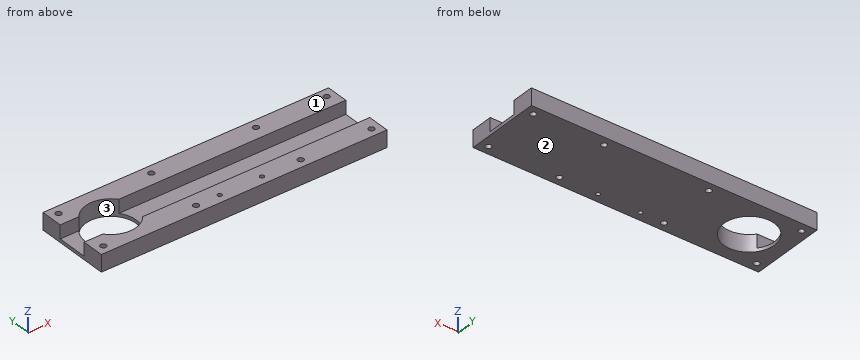
from build123d import *

# Parameters (mm, degrees)
F0_W     = 323.85
F0_H     = 85.09
F1_DEPTH = 19.05
F2_R     = 28.575
F3_DEPTH = 19.051
F4_R     = 3.302
F5_DEPTH = 19.051
F6_R     = 2.413
F7_DEPTH = 19.051
F9_DEPTH = 15.24


with BuildPart() as f1:
    # F0 (on Top) → F1 (new body)
    with BuildSketch(Plane.XY):
        with Locations((161.925, 42.545)):
            Rectangle(F0_W, F0_H)
    extrude(amount=F1_DEPTH)

    # F2 (on face) → F3 (cut, through all)
    with BuildSketch(Plane.XY.offset(19.05)):
        with Locations((43.815, 42.545)):
            Circle(F2_R)
    extrude(amount=-F3_DEPTH, mode=Mode.SUBTRACT)

    # F4 (on face) → F5 (cut, through all)
    with BuildSketch(Plane.XY.offset(19.05)):
        with Locations((9.906, 75.184)):
            Circle(F4_R)
        with Locations((115.062, 75.184)):
            Circle(F4_R)
        with Locations((233.68, 75.184)):
            Circle(F4_R)
        with Locations((313.944, 75.184)):
            Circle(F4_R)
        with Locations((115.062, 9.906)):
            Circle(F4_R)
        with Locations((9.906, 9.906)):
            Circle(F4_R)
        with Locations((233.68, 9.906)):
            Circle(F4_R)
        with Locations((313.944, 9.906)):
            Circle(F4_R)
    extrude(amount=-F5_DEPTH, mode=Mode.SUBTRACT)

    # F6 (on face) → F7 (cut, through all)
    with BuildSketch(Plane.XY.offset(19.05)):
        with Locations((141.859, 10.033)):
            Circle(F6_R)
        with Locations((189.865, 10.033)):
            Circle(F6_R)
    extrude(amount=-F7_DEPTH, mode=Mode.SUBTRACT)

    # F8 (on face) → F9 (cut)
    with BuildSketch(Plane.XY.offset(19.05)):
        with BuildLine():
            Line((323.85, 60.0075), (66.433393, 60.0075))
            ThreePointArc((66.433393, 60.0075), (70.859881, 51.770238), (72.39, 42.545))
            ThreePointArc((72.39, 42.545), (70.859881, 33.319762), (66.433393, 25.0825))
            Line((66.433393, 25.0825), (323.85, 25.0825))
            Line((323.85, 25.0825), (323.85, 60.0075))
        make_face()
        with BuildLine():
            Line((21.196607, 60.0075), (0, 60.0075))
            Line((0, 60.0075), (0, 25.0825))
            Line((0, 25.0825), (21.196607, 25.0825))
            ThreePointArc((21.196607, 25.0825), (15.24, 42.545), (21.196607, 60.0075))
        make_face()
    extrude(amount=-F9_DEPTH, mode=Mode.SUBTRACT)


solid = f1.part
Verification items for the finished model (mm, model axes). Face numbers are marked on the shaded views. Coordinates: 2 decimals unless noted, no trailing zeros. Order: outer loops, then holes, each group sorted by start corner. A loop starts at its lowest first (then second) coordinate and runs counter-clockwise, first axis right, second up. Notation, with made-up numbers: M 66.25,17.5 L 115.25,17.5 A15 ccw 115.25,35.5 Z; hole C -27.5,33.5 d4. An arc over 180 degrees is marked long. One line per item, written item: value. Start each with the question number.
Item 1: Sectioned sample at A-A on z = 16. Give the number of separate pieces and of enclosed holes in the cut face, then the cut area to 3 significant figures.
Item 2: Sectioned sample at C-C on y = 67. Record the cut outline in (x, z), then the cut area to 3 significant figures.
Item 3: Sectioned sample at D-D on x = 296. Record the cut outline in (y, z), then the cut area to 3 significant figures.
Item 4: Mould release check, pull along Z, two halves, no side actions. Record for the marked faces 1, 2 and 3: pulls with the +Z half, pulls with the -Z half, needs draft (parallel to the pull), parting line crosses it, or undercut.
Item 5: Depth check by flat-ended pin: P1, Ø10.5, axis at x = 115.062, y = 9.906, coming from the -Z side; P2, Ø5.5, axis at x = 115.062, y = 75.184, coming from the +Z side. Enter the tip coordinate at first touch or a pass-through.
Item 6: Sectioned sample at B-B on x = 233.68. Record the cut outline in (y, z), then the cut area to 3 significant figures.
Item 7: Thickness scan on probe 1 along Y at (x, z) = (115, 15); probe 2 along X at (y, z) = (25, 7.25); probe 3 along Y at (x, z) = (128.5, 5.75). Record the ranges inside material, lowest first.
Calculated:
1. separate pieces: 2
1. enclosed holes: 10
1. area: 15,200 mm^2
2. outline: M 0,0 L 29.03,0 L 29.03,19.05 L 0,19.05 Z; M 58.6,0 L 323.85,0 L 323.85,19.05 L 58.6,19.05 Z
2. area: 5,610 mm^2
3. outline: M 0,0 L 85.09,0 L 85.09,19.05 L 60.01,19.05 L 60.01,3.81 L 25.08,3.81 L 25.08,19.05 L 0,19.05 Z
3. area: 1,090 mm^2
4. face 1: pulls with the +Z half
4. face 2: pulls with the -Z half
4. face 3: needs draft
5. P1: z = 0
5. P2: through
6. outline: M 0,0 L 6.6,0 L 6.6,19.05 L 0,19.05 Z; M 13.21,0 L 71.88,0 L 71.88,19.05 L 60.01,19.05 L 60.01,3.81 L 25.08,3.81 L 25.08,19.05 L 13.21,19.05 Z; M 78.49,0 L 85.09,0 L 85.09,19.05 L 78.49,19.05 Z
6. area: 837 mm^2
7. probe 1: 0 to 6.6, 13.21 to 25.08, 60.01 to 71.88, 78.49 to 85.09
7. probe 2: 0 to 21.26, 66.37 to 323.85
7. probe 3: 0 to 25.08, 60.01 to 85.09
